```python
from build123d import *

# Parameters (mm, degrees)
TOOTHCUT_DEPTH  = 33.511421565
TEETHCUTS_COUNT = 9
TEETHCUTS_ANGLE = 320
BORSKE_R        = 5
BORE_DEPTH      = 50.0005
KEYSKE_W        = 4
KEYSKE_H        = 6.8
KEYWAY_DEPTH    = 50.0005


with BuildPart() as part:
    # BasProSke → Base-Revolve (revolve)
    with BuildSketch(Plane(origin=(0, 0, 0), x_dir=(1, 0, 0), z_dir=(0, 1, 0)), mode=Mode.PRIVATE) as base_revolve_sk:
        with BuildLine():
            Line((0, 0), (0, 18.285742546))
            ThreePointArc((0, 18.285742546), (0.191950592, 20.485447071), (0.762, 22.618657961))
            Line((0.762, 22.618657961), (5.0505, 22.618657961))
            ThreePointArc((5.0505, 22.618657961), (5.620549408, 20.485447071), (5.8125, 18.285742546))
            Line((5.8125, 18.285742546), (5.8125, 0))
            Line((5.8125, 0), (0, 0))
        make_face()
    revolve(base_revolve_sk.sketch.rotate(Axis((-10, 0, 0), (1, 0, 0)), 180), axis=Axis((-10, 0, 0), (1, 0, 0)))

    # TooCutSke → ToothCut (cut, through all)
    with BuildSketch(Plane(origin=(0, 0, 0), x_dir=(0, 0, -1), z_dir=(1, 0, 0))):
        with BuildLine():
            ThreePointArc((3.55621581, 16.946717295), (5.415747479, 19.676223939), (8.046347206, 21.673224093))
            ThreePointArc((8.046347206, 21.673224093), (0, 23.118657961), (-8.046347206, 21.673224093))
            ThreePointArc((-8.046347206, 21.673224093), (-5.415747479, 19.676223939), (-3.55621581, 16.946717295))
            ThreePointArc((-3.55621581, 16.946717295), (0, 14.681157961), (3.55621581, 16.946717295))
        make_face()
    toothcut = extrude(amount=TOOTHCUT_DEPTH, mode=Mode.SUBTRACT)

    # TeethCuts: ToothCut ×9 about axis
    teethcuts_axis = Axis((-10, 0, 0), (1, 0, 0))
    for i in range(1, TEETHCUTS_COUNT):
        add(toothcut.rotate(teethcuts_axis, i * TEETHCUTS_ANGLE / (TEETHCUTS_COUNT - 1)), mode=Mode.SUBTRACT)

    # BorSke → Bore (cut, symmetric)
    with BuildSketch(Plane(origin=(0, 0, 0), x_dir=(0, 0, -1), z_dir=(1, 0, 0))):
        with Locations(Location((0, 0, 0), (0, 0, 180))):
            Circle(BORSKE_R)
    extrude(amount=BORE_DEPTH, both=True, mode=Mode.SUBTRACT)

    # KeySke → Keyway (cut, symmetric)
    with BuildSketch(Plane(origin=(0, 0, 0), x_dir=(0, 0, -1), z_dir=(1, 0, 0))):
        with Locations((0, 3.4)):
            Rectangle(KEYSKE_W, KEYSKE_H)
    extrude(amount=KEYWAY_DEPTH, both=True, mode=Mode.SUBTRACT)


solid = part.part
```
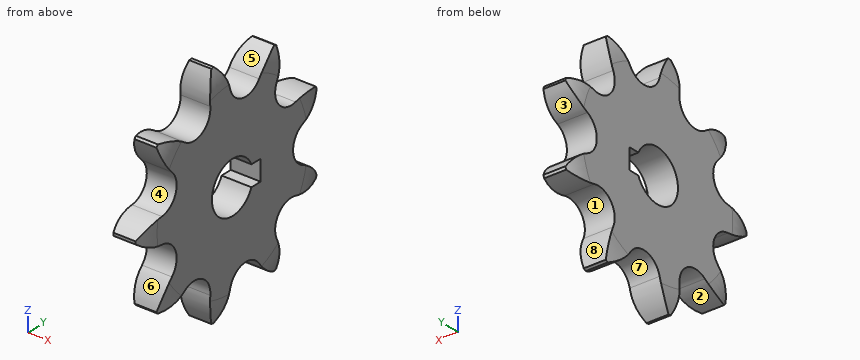
Part model, mm, in its own coordinate system. Face numbers are marked on the shaded views. A direction names the side the tool comes from. Coordinates: 2 decimals unless noted, no trailing zeros. Order: outer loops, then holes, each group sorted by start corner. A loop starts at its lowest first (then second) coordinate and runs counter-clockwise, first axis right, second up. Notation, with made-up numbers: (37.5, 60) - (95.5, 60) arc R16 cw to (95.5, 78) - close; hole circle Ø2 at (80.5, 33). An arc over 180 degrees is marked (long way). Return JSON: item names as keys, results as strings. Group by question number.
Item 1: Cut at C-C (y = -7.5). List the corners of the cut face in (x, z).
Item 2: Which spindle directions (+Z, -Z, +X, -X, +Y, -Y) get a long thin tool onto all of the face, cutting with end or side? Do the marked faces 1, 2, 3, 4 and 5. Say none if no direction does.
Item 3: Pin check, flat tips, straight feed: pin 1 (2.5 mm diameter, centred on x = 2, y = 5.5, fed in from +Z); pin 2 (3 mm diameter, centred on x = 1.5, z = -11, fed in from -Y); pin 3 (1.2 mm diameter, centred on x = 1.5, z = -1, fed in from -Y). Stop position of each tip, or through.
Item 4: Cut at A-A (y = 2). List the corners of the cut face in (x, z), plus the area to 3 significant figures.
Item 5: Drill centre lines: probe 1 along Y at (x, z) = (4.6, 1.5); probe 2 along Z at (x, y) = (1.65, 0); probe 3 along Z at (x, y) = (0.5, -2). Where is each one in solid material? Low to high. Write a range as from..to.
Item 6: Cut at B-B (y = 14). List the corners of the cut face in (x, z), plus the area to 3 significant figures.
Item 7: Pull direction Y, two halves, no side cores. Call the marked faces 6, 7 and 8: pulls with the +Y half, pulls with the -Y half, needs draft (parallel to the pull), parting line crosses it, or undercut.
Check values:
{
 "1": {"outline": "(0, -12.63) - (5.81, -12.63) - (5.81, 12.63) - (0, 12.63) - close"},
 "2": {"face 1": "+X, -X", "face 2": "-Z, +X, -X", "face 3": "+X, -X, +Y", "face 4": "+X, -X, -Y", "face 5": "+Z, +X, -X"},
 "3": {"pin 1": "stops at z = 16.48", "pin 2": "stops at y = -16.95", "pin 3": "stops at y = -22.46"},
 "4": {"outline": "(0, -14.6) - (5.81, -14.6) - (5.81, -4.58) - (0, -4.58) - close; (0, 4.58) - (5.81, 4.58) - (5.81, 14.6) - (0, 14.6) - close", "area": "116 mm2"},
 "5": {"probe 1": "y = -20.65..-4.77, 6.8..14.98", "probe 2": "z = -16.1..-5, 5..16.1", "probe 3": "z = -20.44..-4.58, 4.58..20.44"},
 "6": {"outline": "(0, -8.04) - (5.81, -8.04) - (5.81, 8.04) - (0, 8.04) - close", "area": "93.5 mm2"},
 "7": {"face 6": "pulls with the -Y half", "face 7": "undercut", "face 8": "pulls with the +Y half"}
}
